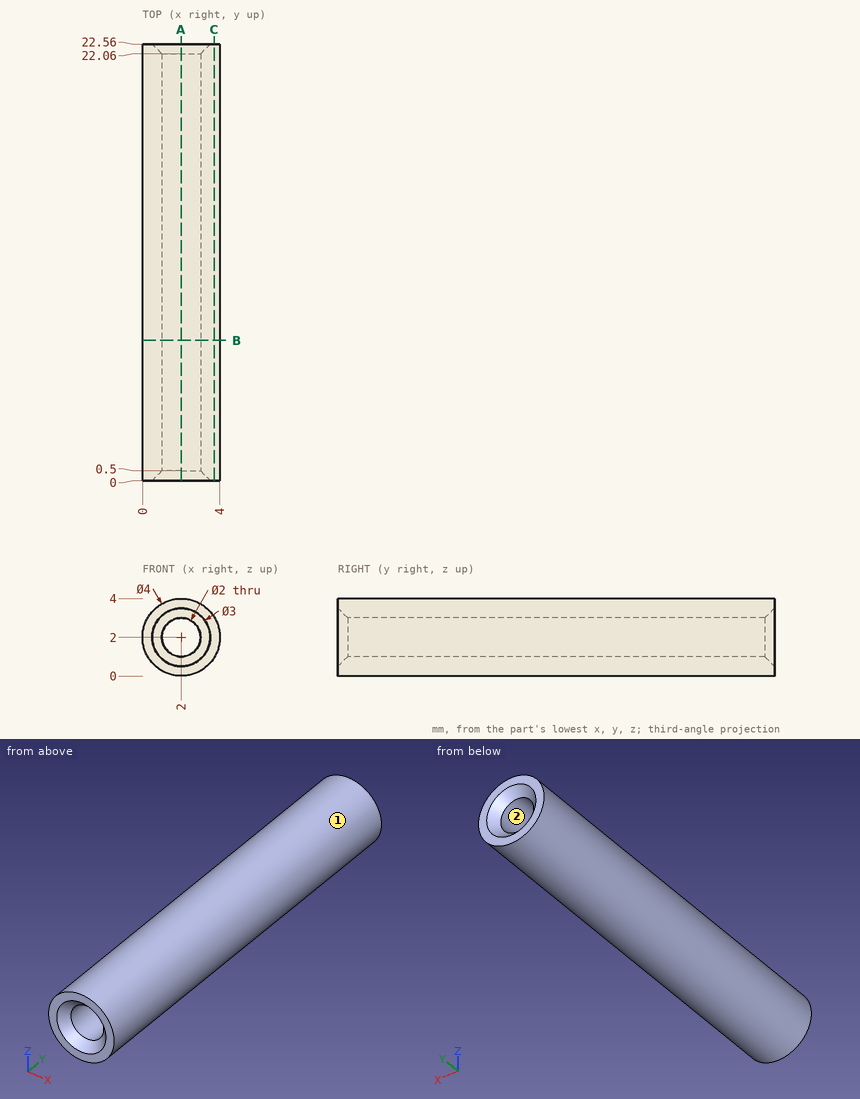
Geometry: see drawing. Coordinates: mm, zero at the bounding-box minimum. Coordinates: 2 decimals unless noted, no trailing zeros. Write each loop counter-clockwise with the first axis right and the second up, starting at its lowest first coordinate (ties: lowest second). Pieces come first, ordered by that corner, then holes.
1) Section C-C on x = 3.7. Output: boundary loops of the cut face in (y, z).
2) Material intervals for line 1 along Z through (x, y) = (2, 8); line 2 along X through (y, z) = (14, 1.9); line 3 along Z through (x, y) = (2.7, 7.75), sorted ascending.
3) Section A-A on x = 2. Output: boundary loops of the cut face in (y, z), and give its area (3 significant figures).
4) Section B-B on y = 7.25. Output: boundary loops of the cut face in (x, z).
5) Mould query, pull axis Z, two halves, no side actions, for the marked faces 1 and 2. Classes: pulls with the +Z half, pulls with the -Z half, needs draft (parallel to the pull), parting line crosses it, or undercut.
Check result:
1. outline: (0, 0.95) - (22.56, 0.95) - (22.56, 3.05) - (0, 3.05) - close
2. line 1: z = 0 to 1, 3 to 4
2. line 2: x = 0 to 1.01, 2.99 to 4
2. line 3: z = 0.13 to 1.29, 2.71 to 3.87
3. outline: (0, 0) - (22.56, 0) - (22.56, 0.5) - (22.06, 1) - (0.5, 1) - (0, 0.5) - close; (0, 3.5) - (0.5, 3) - (22.06, 3) - (22.56, 3.5) - (22.56, 4) - (0, 4) - close
3. area: 44.6 mm2
4. outline: circle Ø4 at (2, 2); hole circle Ø2 at (2, 2)
5. face 1: parting line crosses it
5. face 2: undercut
